```python
from build123d import *

# Parameters (mm, degrees)
F0_R     = 1
F1_DEPTH = 2


with BuildPart() as f1:
    # F0 (on Front) → F1 (new body)
    with BuildSketch(Plane.XZ):
        with BuildLine():
            Line((14.785155, 3.270633), (4.98624, 24.321079))
            ThreePointArc((4.98624, 24.321079), (2.956693, 26.637668), (0, 27.5))
            ThreePointArc((0, 27.5), (-2.956693, 26.637668), (-4.98624, 24.321079))
            Line((-4.98624, 24.321079), (-14.785155, 3.270633))
            ThreePointArc((-14.785155, 3.270633), (-14.639389, 1.063565), (-12.7, 0))
            Line((-12.7, 0), (0, 0))
            Line((0, 0), (12.7, 0))
            ThreePointArc((12.7, 0), (14.639389, 1.063565), (14.785155, 3.270633))
        make_face()
        with Locations((-12.7, 2.3)):
            Circle(F0_R, mode=Mode.SUBTRACT)
        with Locations((12.7, 2.3)):
            Circle(F0_R, mode=Mode.SUBTRACT)
        with BuildLine():
            ThreePointArc((0, 25), (3, 22), (0, 19))
            ThreePointArc((0, 19), (-3, 22), (0, 25))
        make_face(mode=Mode.SUBTRACT)
    extrude(amount=F1_DEPTH)


solid = f1.part
```
Part model, mm, in its own coordinate system. Round coordinates to 2 decimals unless told otherwise and drop trailing zeros. Loops run counter-clockwise (first coordinate to the right, second up) from the corner with the lowest first, then second, coordinate; pieces in that order, holes last.
1. Flat gauge pin, fed straight in: pin 1 (10 mm diameter, centred on x = -2.5, z = 12.5, fed in from +Y). Where does the tip first touch, or does it go through?
Solutions:
pin 1: stops at y = 0
2. Slice it at B-B (y = -1.3). Give the cut face in (x, z), and give its area (3 significant figures).
Solutions:
outline: (-14.79, 3.27) arc R2.3 ccw to (-12.7, 0) - (12.7, 0) arc R2.3 ccw to (14.79, 3.27) - (4.99, 24.32) arc R5.5 ccw to (-4.99, 24.32) - close; hole circle Ø2 at (-12.7, 2.3); hole circle Ø6 at (0, 22); hole circle Ø2 at (12.7, 2.3)
area: 500 mm2
3. Two-plate mould, pull along Z, no slides. Class faces 1 (the face through (0, -2, 11)), 2 (the face through (-14.657, -0.986, 1.091)), 3 (the face through (-11.746, -0.986, 2.6)): pulls with the +Z half, pulls with the -Z half, needs draft (parallel to the pull), parting line crosses it, or undercut.
Solutions:
face 1: needs draft
face 2: parting line crosses it
face 3: undercut
4. Slice it at A-A (z = 2.3). Give the cut face in (x, y), and give its area (3 significant figures).
Solutions:
outline: (-15, -2) - (-13.7, -2) - (-13.7, 0) - (-15, 0) - close; (-11.7, -2) - (11.7, -2) - (11.7, 0) - (-11.7, 0) - close; (13.7, -2) - (15, -2) - (15, 0) - (13.7, 0) - close
area: 52.0 mm2
5. Slice it at D-D (z = 22). Give the cut face in (x, y).
Solutions:
outline: (-6.07, -2) - (-3, -2) - (-3, 0) - (-6.07, 0) - close; (3, -2) - (6.07, -2) - (6.07, 0) - (3, 0) - close
6. Slice it at C-C (x = 0.5). Give the cut face in (y, z).
Solutions:
outline: (-2, 0) - (0, 0) - (0, 19.04) - (-2, 19.04) - close; (-2, 24.96) - (0, 24.96) - (0, 27.48) - (-2, 27.48) - close
7. Drill centre lines: line 1 along X through (y, z) = (-1.05, 2.5); line 2 along Z through (x, y) = (12.7, -0.5); line 3 along Z through (x, y) = (12, -1.65). Where is each one in solid material? Low to high.
Solutions:
line 1: x = -14.99 to -13.68, -11.72 to 11.72, 13.68 to 14.99
line 2: z = 0 to 1.3, 3.3 to 7.75
line 3: z = 0 to 1.59, 3.01 to 9.25
